Read the model definition and answer for the solid it produces. Units are mm, in the model's axes. A direction names the side the tool comes from. Round coordinates to 2 decimals unless told otherwise and drop trailing zeros. Order: outer loops, then holes, each group sorted by start corner. A loop starts at its lowest first (then second) coordinate and runs counter-clockwise, first axis right, second up. Notation, with made-up numbers: (20.5, 76.5) -> (73.5, 76.5) arc R13 ccw to (73.5, 98.5) -> close; hole circle Ø7 at (67, 64.25). An arc over 180 degrees is marked (long way). Use a Markdown table: item, result. Add a question column.
1. Section C-C, the plane y = 2.3 is taken. Give the number of separate pieces and of enclosed holes in the cut face, then the cut area to 3 significant figures.
2. Consider L1, parallel to X at y = 2.35, z = 0; L2, parallel to X at y = 1, z = -28.5; L3, parallel to X at y = 0.35, z = -31.5. Determine where each line is inside the solid, lowest interval first. Write a range as [from, to].
3. Given pin 1 (1.9 mm diameter, centred on x = 159.5, z = -21.5, fed in from +Y), flat-ended and moving along its own axis, determine where the tip first touches the part or whether it passes through.
4. Section A-A, the plane z = 0 is taken. Give the vertices of the cut face in (x, y).
5. Section B-B, the plane x = 225 is taken. Give the vertices of the cut face in (y, z).
6. For faces 4 (the face through (280.777, 0.225, 31.922)), 5 (the face through (152, 3.6, -1)), 6 (the face through (156, 0.6, 12)), determine the directions among +Z, -Z, +X, -X, +Y, -Y from which every point of the face is accessible in a straight line to the end or side of a thin tool.
7. The mould has two halves that part along X. Classify faces 1 (the face through (150, 1.8, -0.5)), 2 (the face through (217.1, 0, -50.4)), 3 (the face through (277.12, 0.23, 36.41)): +X half, -X half, draft (parallel to the pull), parting line (faces both ways), or undercut.
```python
from build123d import *

# Parameters (mm, degrees)
SKIZZE1_R                       = 50
AUFSATZ_LINEAR_AUSTRAGEN1_DEPTH = 3.6
SCHNITT_LINEAR_AUSTRAGEN1_DEPTH = 3
SCHNITT_LINEAR_AUSTRAGEN2_DEPTH = 300.577355237
SCHNITT_LINEAR_AUSTRAGEN3_DEPTH = 3
FASE1_SIZE                      = 0.6
SCHNITT_LINEAR_AUSTRAGEN4_DEPTH = 300.577355237
AUFSATZ_LINEAR_AUSTRAGEN4_DEPTH = 101.2
AUFSATZ_LINEAR_AUSTRAGEN5_DEPTH = 101.2


with BuildPart() as part:
    # Skizze1 → Aufsatz-Linear austragen1 (new body)
    with BuildSketch(Plane(origin=(0, 0, 0), x_dir=(1, 0, 0), z_dir=(0, 1, 0))):
        with BuildLine():
            Line((280.118489624, 75.05752308), (144.888873943, 38.822856765))
            ThreePointArc((144.888873943, 38.822856765), (150, 0), (144.888873943, -38.822856765))
            Line((144.888873943, -38.822856765), (280.118489624, -75.05752308))
            ThreePointArc((280.118489624, -75.05752308), (290, 0), (280.118489624, 75.05752308))
        make_face()
        with Locations(Location((225, 0, 0), (0, 0, 270))):
            Circle(SKIZZE1_R, mode=Mode.SUBTRACT)
    extrude(amount=AUFSATZ_LINEAR_AUSTRAGEN1_DEPTH)

    # Skizze2 → Schnitt-Linear austragen1 (cut)
    with BuildSketch(Plane(origin=(0, 3.6, 0), x_dir=(1, 0, 0), z_dir=(0, 1, 0))):
        with BuildLine():
            Line((150.587836318, 40.349889131), (153.678798963, 41.178110076))
            ThreePointArc((153.678798963, 41.178110076), (159.1, 0), (153.678798963, -41.178110076))
            Line((153.678798963, -41.178110076), (150.587836318, -40.349889131))
            ThreePointArc((150.587836318, -40.349889131), (155.9, 0), (150.587836318, 40.349889131))
        make_face()
        with BuildLine():
            Line((271.328564605, 72.702269769), (274.419527249, 73.530490714))
            ThreePointArc((274.419527249, 73.530490714), (284.1, 0), (274.419527249, -73.530490714))
            Line((274.419527249, -73.530490714), (271.328564605, -72.702269769))
            ThreePointArc((271.328564605, -72.702269769), (280.9, 0), (271.328564605, 72.702269769))
        make_face()
    extrude(amount=-SCHNITT_LINEAR_AUSTRAGEN1_DEPTH, mode=Mode.SUBTRACT)

    # Skizze3 → Schnitt-Linear austragen2 (cut, through all)
    with BuildSketch(Plane(origin=(0, 3.6, 0), x_dir=(1, 0, 0), z_dir=(0, 1, 0))):
        Polygon((152.525600121, 25.123521005), (158.474269289, 25.906678158), (159.779531212, 15.992229544), (153.830862043, 15.209072391), align=None)
        Polygon((276.456207793, -41.439295032), (282.404876961, -42.222452186), (283.710138883, -32.308003572), (277.761469715, -31.524846419), align=None)
    extrude(amount=-SCHNITT_LINEAR_AUSTRAGEN2_DEPTH, mode=Mode.SUBTRACT)

    # Skizze4 → Schnitt-Linear austragen3 (cut)
    with BuildSketch(Plane(origin=(0, 3.6, 0), x_dir=(1, 0, 0), z_dir=(0, 1, 0))):
        Polygon((150.999552071, 21.392411606), (160.914000685, 22.697673528), (161.305579262, 19.723338944), (151.391130648, 18.418077021), align=None)
        Polygon((275.32173832, -34.733851049), (285.236186933, -36.039112971), (284.844608357, -39.013447555), (274.930159743, -37.708185633), align=None)
    extrude(amount=-SCHNITT_LINEAR_AUSTRAGEN3_DEPTH, mode=Mode.SUBTRACT)

    # Fase1
    fase1_edges = [part.edges().sort_by_distance(p)[0] for p in [
        (225, 0, -50),
    ]]
    chamfer(fase1_edges, length=FASE1_SIZE)

    # Skizze5 → Schnitt-Linear austragen4 (cut, through all)
    with BuildSketch(Plane.XZ):
        Polygon((168.457464105, 45.138041466), (266.209157725, 71.33052883), (268.020891041, 64.569048046), (170.269197421, 38.376560682), align=None)
        Polygon((168.457464105, -45.138041466), (266.209157725, -71.33052883), (268.020891041, -64.569048046), (170.269197421, -38.376560682), align=None)
    extrude(amount=-SCHNITT_LINEAR_AUSTRAGEN4_DEPTH, mode=Mode.SUBTRACT)

    # Skizze6 → Aufsatz-Linear austragen4 (add)
    with BuildSketch(Plane(origin=(168.457464105, 0, 45.138041466), x_dir=(0.25881904510252185, 0, -0.965925826289068), z_dir=(0.9659258262890681, 0, 0.25881904510252185))):
        Polygon((0, 3.6), (7, 3.6), (7, 0), (0, 3), align=None)
    extrude(amount=AUFSATZ_LINEAR_AUSTRAGEN4_DEPTH)

    # Skizze7 → Aufsatz-Linear austragen5 (add)
    with BuildSketch(Plane(origin=(168.457464105, 0, -45.138041466), x_dir=(-0.2588190451025227, 0, -0.9659258262890678), z_dir=(0.9659258262890678, 0, -0.2588190451025227))):
        Polygon((-7, 0), (-7, 3.6), (0, 3.6), (0, 3), align=None)
    extrude(amount=AUFSATZ_LINEAR_AUSTRAGEN5_DEPTH)


solid = part.part
```
Verdict:
| question | item | result |
|---|---|---|
| 1 | separate pieces | 3 |
| 1 | enclosed holes | 1 |
| 1 | area | 7,130 mm2 |
| 2 | L1 | x = [150, 155.9], [159.1, 175], [275, 280.9], [284.1, 290] |
| 2 | L2 | x = [147.27, 153.27], [156.53, 183.92], [266.08, 279.45], [282.67, 288.6] |
| 2 | L3 | x = [146.66, 185.85], [264.15, 288.28] |
| 3 | pin 1 | stops at y = 0.6 |
| 4 | outline | (150, 0) -> (174.4, 0) -> (175, 0.6) -> (175, 3.6) -> (159.1, 3.6) -> (159.1, 0.6) -> (155.9, 0.6) -> (155.9, 3.6) -> (150, 3.6) -> close; (275, 0.6) -> (275.6, 0) -> (290, 0) -> (290, 3.6) -> (284.1, 3.6) -> (284.1, 0.6) -> (280.9, 0.6) -> (280.9, 3.6) -> (275, 3.6) -> close |
| 5 | outline | (0, -53.04) -> (3, -60.29) -> (3.6, -60.29) -> (3.6, -50) -> (0.6, -50) -> (0, -50.6) -> close; (0, 50.6) -> (0.6, 50) -> (3.6, 50) -> (3.6, 60.29) -> (3, 60.29) -> (0, 53.04) -> close |
| 6 | face 4 | +Y, -Y |
| 6 | face 5 | +Z, -Z, +X, -X, +Y |
| 6 | face 6 | +Y |
| 7 | face 1 | -X half |
| 7 | face 2 | draft |
| 7 | face 3 | undercut |
